```python
from build123d import *

# Parameters (mm, degrees)
SKETCH1_W           = 100
SKETCH1_H           = 100
BOSS_EXTRUDE1_DEPTH = 20
SKETCH2_W           = 92
SKETCH2_H           = 92
CUT_EXTRUDE1_DEPTH  = 16
FILLET1_R           = 2
SKETCH3_R           = 6
SKETCH3_R_2         = 2.713966801
CUT_EXTRUDE2_DEPTH  = 16


with BuildPart() as part:
    # Sketch1 → Boss-Extrude1 (new body)
    with BuildSketch(Plane.XY):
        Rectangle(SKETCH1_W, SKETCH1_H)
    extrude(amount=BOSS_EXTRUDE1_DEPTH)

    # Sketch2 → Cut-Extrude1 (cut)
    with BuildSketch(Plane.XY.offset(20)):
        Rectangle(SKETCH2_W, SKETCH2_H)
    extrude(amount=-CUT_EXTRUDE1_DEPTH, mode=Mode.SUBTRACT)

    # Fillet1
    fillet1_edges = [part.edges().sort_by_distance(p)[0] for p in [
        (-46, -46, 12),
        (-46, 46, 12),
        (46, 46, 12),
        (46, -46, 12),
        (-50, 50, 10),
        (50, 50, 10),
        (50, -50, 10),
        (-50, -50, 10),
    ]]
    fillet(fillet1_edges, radius=FILLET1_R)

    # Sketch3 → Cut-Extrude2 (cut)
    with BuildSketch(Plane.XY):
        Circle(SKETCH3_R)
        with Locations((-40, 40)):
            Circle(SKETCH3_R_2)
        with Locations((40, 40)):
            Circle(SKETCH3_R_2)
        with Locations((40, -40)):
            Circle(SKETCH3_R_2)
        with Locations((-40, -40)):
            Circle(SKETCH3_R_2)
    extrude(amount=CUT_EXTRUDE2_DEPTH, mode=Mode.SUBTRACT)


solid = part.part
```
Here's how the part is built. I have some questions about the finished solid (model axes, mm). A direction names the side the tool comes from. Coordinates: 2 decimals unless noted, no trailing zeros. Loops run counter-clockwise (first coordinate to the right, second up) from the corner with the lowest first, then second, coordinate; pieces in that order, holes last. Notation, with made-up numbers: (-36.75, -34) -> (19.25, -34) arc R36 cw to (19.25, 4) -> close; hole circle Ø9 at (71.5, -29). An arc over 180 degrees is marked (long way). Return JSON: item names as keys, results as strings.
1) Thinking about a two-plate mould opening in X: for faces 1 (the face through (-50, -1, 10)), 2 (the face through (-46, -1, 12)), 3 (the face through (-1, 12, 0)), which applies, +X half, -X half, draft (parallel to the pull), parting line (faces both ways), or undercut?
Results below:
{"face 1": "-X half", "face 2": "undercut", "face 3": "draft"}
2) I need wall thicknesses on line 1 (X direction, y = -40, z = 2.05); line 2 (X direction, y = -18, z = 10.25). Which ranges of each line are inside material? Lowest first, please. Write a range as from..to.
Results below:
{"line 1": "-50..-42.71, -37.29..37.29, 42.71..50", "line 2": "-50..-46, 46..50"}
3) If we section it at B-B, the plane y = 0: Write out the boundary of the cut face in (x, z).
Results below:
{"outline": "(-50, 0) -> (-6, 0) -> (-6, 4) -> (-46, 4) -> (-46, 20) -> (-50, 20) -> close; (6, 0) -> (50, 0) -> (50, 20) -> (46, 20) -> (46, 4) -> (6, 4) -> close"}
4) Will these pins go through, and if not, where does the flat tip stop? pin 1 (4.5 mm diameter, centred on x = 40, y = -40, fed in from +Z); pin 2 (5 mm diameter, centred on x = -8, y = 14, fed in from +Z).
Results below:
{"pin 1": "through", "pin 2": "z = 4"}
5) For faces 4 (the face through (46, -1, 12)), 5 (the face through (-6, 0, 2)), which set-ups out of +Z, -Z, +X, -X, +Y, -Y let a thin tool reach every point of the face, with its end or its side?
Results below:
{"face 4": "+Z", "face 5": "+Z, -Z"}
6) If we section it at A-A, the plane x = -40: Write out the boundary of the cut face in (y, z).
Results below:
{"outline": "(-50, 0) -> (-42.71, 0) -> (-42.71, 4) -> (-46, 4) -> (-46, 20) -> (-50, 20) -> close; (-37.29, 0) -> (37.29, 0) -> (37.29, 4) -> (-37.29, 4) -> close; (42.71, 0) -> (50, 0) -> (50, 20) -> (46, 20) -> (46, 4) -> (42.71, 4) -> close"}
7) If we section it at C-C, the plane z = 14.25: Write out the boundary of the cut face in (x, y), then the cut area to 3 significant figures.
Results below:
{"outline": "(-50, -48) arc R2 ccw to (-48, -50) -> (48, -50) arc R2 ccw to (50, -48) -> (50, 48) arc R2 ccw to (48, 50) -> (-48, 50) arc R2 ccw to (-50, 48) -> close; hole (-46, -44) arc R2 ccw to (-44, -46) -> (44, -46) arc R2 ccw to (46, -44) -> (46, 44) arc R2 ccw to (44, 46) -> (-44, 46) arc R2 ccw to (-46, 44) -> close", "area": "1,540 mm²"}
